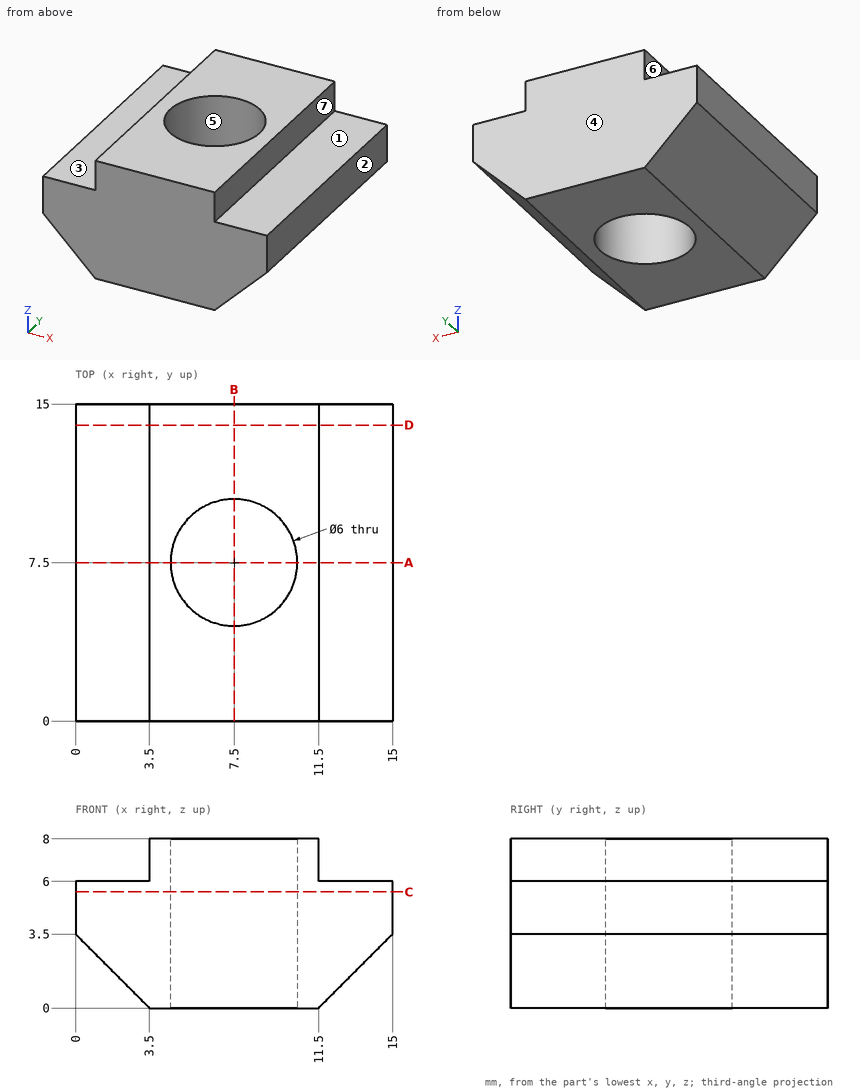
Check sheet for the drawn part. Datum: minimum x, y, z corner. Units: mm. A direction names the side the tool comes from. Coordinates: 2 decimals unless noted, no trailing zeros. Order: outer loops, then holes, each group sorted by start corner. A loop starts at its lowest first (then second) coordinate and runs counter-clockwise, first axis right, second up. Notation, with made-up numbers: (27, 56.5) -> (62, 56.5) arc R20 cw to (62, 81.5) -> close; hole circle Ø10 at (-5, 54). An arc over 180 degrees is marked (long way). Use a Markdown table: item, result. Add a question column.
1. Set-up check for the marked faces 1, 2 and 3: record each of +Z, -Z, +X, -X, +Y, -Y from which the full face is reachable in a straight line by a thin tool's end or side.
2. Cross-section at D-D (y = 14). Enter the section's corners in (x, z).
3. Cross-section at A-A (y = 7.5). Enter the section's corners in (x, z).
4. Material ranges on L1, parallel to Y at x = 7.5, z = 5; L2, parallel to X at y = 11.5, z = 7; L3, parallel to X at y = 9.75, z = 1.75, recorded low to high.
5. Cross-section at B-B (x = 7.5). Enter the section's corners in (y, z).
6. Mould release check, pull along X, two halves, no side actions. Record for the marked faces 4, 5, 6 and 7: pulls with the +X half, pulls with the -X half, needs draft (parallel to the pull), parting line crosses it, or undercut.
7. Go/stop test with flat-tipped pins: pin 1 Ø5 at (x, y) = (7.5, 7.5) entering from -Z; pin 2 Ø0.6 at (y, z) = (7, 7) entering from +X; pin 3 Ø3 at (x, y) = (1.5, 9) entering from +Z. Record where each tip stops, or that it passes through.
8. Cross-section at C-C (z = 5.5). Enter the section's corners in (x, y), and give its area (3 significant figures).
Filled sheet:
| question | item | result |
|---|---|---|
| 1 | face 1 | +Z, +X, +Y, -Y |
| 1 | face 2 | +Z, -Z, +X, +Y, -Y |
| 1 | face 3 | +Z, -X, +Y, -Y |
| 2 | outline | (0, 3.5) -> (3.5, 0) -> (11.5, 0) -> (15, 3.5) -> (15, 6) -> (11.5, 6) -> (11.5, 8) -> (3.5, 8) -> (3.5, 6) -> (0, 6) -> close |
| 3 | outline | (0, 3.5) -> (3.5, 0) -> (4.5, 0) -> (4.5, 8) -> (3.5, 8) -> (3.5, 6) -> (0, 6) -> close; (10.5, 0) -> (11.5, 0) -> (15, 3.5) -> (15, 6) -> (11.5, 6) -> (11.5, 8) -> (10.5, 8) -> close |
| 4 | L1 | 0 to 4.5, 10.5 to 15 |
| 4 | L2 | 3.5 to 11.5 |
| 4 | L3 | 1.75 to 5.52, 9.48 to 13.25 |
| 5 | outline | (0, 0) -> (4.5, 0) -> (4.5, 8) -> (0, 8) -> close; (10.5, 0) -> (15, 0) -> (15, 8) -> (10.5, 8) -> close |
| 6 | face 4 | needs draft |
| 6 | face 5 | undercut |
| 6 | face 6 | pulls with the -X half |
| 6 | face 7 | pulls with the +X half |
| 7 | pin 1 | through |
| 7 | pin 2 | x = 11.5 |
| 7 | pin 3 | z = 6 |
| 8 | outline | (0, 0) -> (15, 0) -> (15, 15) -> (0, 15) -> close; hole circle Ø6 at (7.5, 7.5) |
| 8 | area | 197 mm2 |
